Geometry: final body of the model. Coordinates: model frame, mm. Face numbers are marked on the shaded views. Coordinates: 2 decimals unless noted, no trailing zeros. Write each loop counter-clockwise with the first axis right and the second up, starting at its lowest first coordinate (ties: lowest second). Pieces come first, ordered by that corner, then holes. Notation, with made-up numbers: M 61.25,7 L 85.25,7 A11 cw 85.25,26 Z; hole C 70,-11 d4. An arc over 180 degrees is marked long. Write item = value, one per line. Start each with the question number.
Item 1: Ray query, L1, parallel to Y at x = 5.2, z = -20; L2, parallel to Z at x = 3.6, y = 12; L3, parallel to X at y = 38, z = -91.5. Return the intervals inside material, ascending. Write a range as [from, to].
Item 2: Section A-A on y = 24.5. Output: boundary loops of the cut face in (x, z).
Item 3: Pull-direction query (Y, two-part tool) for the marked faces 1 and 2; classes: +Y half, -Y half, draft (parallel to the pull), parting line (faces both ways), or undercut.
Item 4: Section C-C on z = -64.5. Output: boundary loops of the cut face in (x, y), plus the area to 3 significant figures.
Item 5: First-contact query: pin 1 Ø3 at (x, z) = (4.5, -73) entering from -Y; pin 2 Ø2 at (x, z) = (3.5, -72.5) entering from +Y; pin 3 Ø3 at (x, y) = (4, 39) entering from +Z. Flat tips, straight axial feed; report the tip coordinate or a pass-through.
Item 6: Section B-B on x = 3. Output: boundary loops of the cut face in (y, z).
Autodesk Inventor part; units mm, degrees
ref_plane "YZ Plane" through (0, 0, 0) normal (1, 0, 0) x (0, 1, 0)
ref_plane "XZ Plane" through (0, 0, 0) normal (0, 1, 0) x (-1, 0, 0)
ref_plane "XY Plane" through (0, 0, 0) normal (0, 0, 1) x (1, 0, 0)
sketch "Náčrt1" plane through (0, 0, 0) normal (1, 0, 0) x (0, 1, 0)
  line L0 (0, 0) -> (100, 0)
  line L1 (100, 0) -> (100, -100)
  line L2 (100, -100) -> (0, -100)
  line L3 (0, -100) -> (0, 0)
  dimension "d0" = 100
  dimension "d1" = 100
extrude "Vysunutí1" add sketch "Náčrt1" along normal blind 2
sketch "Náčrt2" plane through (2, 0, 0) normal (1, 0, 0) x (0, 0, -1)
  line L0 (0, 100) -> (0, 0)
  line L1 (0, 0) -> (100, 0)
  line L2 (100, 0) -> (100, 100)
  line L3 (100, 100) -> (0, 100)
  line L4 (2, 98) -> (2, 2)
  line L5 (2, 2) -> (98, 2)
  line L6 (98, 2) -> (98, 98)
  line L7 (98, 98) -> (2, 98)
  line L8 (4, 96) -> (4, 4)
  line L9 (4, 4) -> (96, 4)
  line L10 (96, 4) -> (96, 96)
  line L11 (96, 96) -> (4, 96)
  dimension "d4" = 2
  dimension "d5" = 2
extrude "Vysunutí2" add sketch "Náčrt2" along normal blind 4 contours L7 L6 L5 L4
properties part number "Zadní kryt"
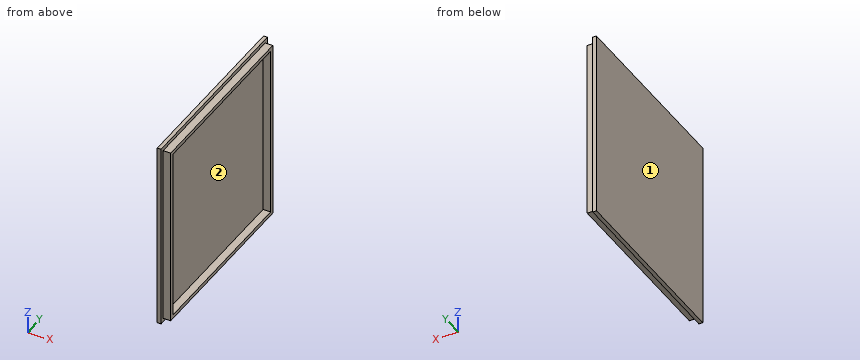
Responses:
q1.L1 = [2, 4], [96, 98]
q1.L2 = [-98, -96], [-4, -2]
q1.L3 = [0, 2]
q2.outline = M 0,-100 L 2,-100 L 2,-98 L 6,-98 L 6,-96 L 2,-96 L 2,-4 L 6,-4 L 6,-2 L 2,-2 L 2,0 L 0,0 Z
q3.face_1 = draft
q3.face_2 = undercut
q4.outline = M 0,0 L 2,0 L 2,2 L 6,2 L 6,4 L 2,4 L 2,96 L 6,96 L 6,98 L 2,98 L 2,100 L 0,100 Z
q4.area = 216 mm²
q5.pin_1 = 2
q5.pin_2 = 98
q5.pin_3 = -2
q6.outline = M 2,-98 L 98,-98 L 98,-2 L 2,-2 Z; hole M 4,-96 L 96,-96 L 96,-4 L 4,-4 Z
